Here's how the part is built. I have some questions about the finished solid (model axes, mm). A direction names the side the tool comes from. Coordinates: 2 decimals unless noted, no trailing zeros. Order: outer loops, then holes, each group sorted by start corner. A loop starts at its lowest first (then second) coordinate and runs counter-clockwise, first axis right, second up. Notation, with made-up numbers: (-13, 63) - (-1, 63) arc R23 ccw to (-1, 82) - close; hole circle Ø2 at (-33, 86). An arc over 180 degrees is marked (long way). Answer in a Markdown table with one row per item. Add a question column.
Item 1: Thinking about a two-plate mould opening in X: for faces 3 (the flat face through (-13, -2, 0)), 4 (the cylindrical face through (-46.344, -13.041, 49.042)), 5 (the cylindrical face through (-12.55, 7.497, 36.005)), which applies, +X half, -X half, draft (parallel to the pull), parting line (faces both ways), or undercut?
Item 2: On a 3-axis mill with a long thin cutter (end or side, diameter ignored), from which of +Z, -Z, +X, -X, +Y, -Y can I reach the whole of each face in a straight line? I mean faces 1 (the flat face through (-47.77, 5, 26)), 2 (the flat face through (-13, -5, 6)). Say none if no direction works.
Item 3: I want a section at C-C (x = -3.5). Please give me the cut outline in (y, z).
Item 4: I want a section at D-D (y = 3). Please give me the cut outline in (x, z).
Item 5: If I drill on line 1 along X through (y, z) = (-9.25, 49.5); line 2 along Z through (x, y) = (-22, -12.25); line 3 along Y through (x, z) = (-42.5, 47), over which ranges is the centre line in solid material (lowest first)? Write a range as from..to.
Item 6: I want a section at A-A (z = 11). Please give me the cut outline in (x, y), plus the area to 3 significant figures.
Item 7: Will these pins go through, and if not, where does the flat tip stop? pin 1 Ø1.5 at (y, z) = (3, 34) entering from -X; pin 2 Ø6 at (x, y) = (-42.77, -9.54) entering from -Z; pin 3 Ø10 at (x, z) = (4, 36) entering from -Y.
Item 8: I want a section at B-B (y = -10.5). Please give me the cut outline in (x, z).
```python
from build123d import *

# Parameters (mm, degrees)
SKETCH_1_W          = 70
SKETCH_1_H          = 25
SKETCH_1_R          = 2.5
EXTRUDE_1_DEPTH     = 52
FILLET_6_R          = 5
FILLET_7_R          = 5
SKETCH_2_W          = 40
SKETCH_2_H          = 19
CUT_EXTRUDE_2_DEPTH = 89.405565637
SKETCH_3_R          = 5
CUT_EXTRUDE_3_DEPTH = 75.906573986


with BuildPart() as part:
    # 草图1 → 凸台-拉伸1 (new body)
    with BuildSketch(Plane.XY):
        with Locations((-12.770229498, -2.044553468)):
            Rectangle(SKETCH_1_W, SKETCH_1_H)
        with Locations(Location((-42.770229498, -9.544553468, 0), (0, 0, 180))):
            Circle(SKETCH_1_R, mode=Mode.SUBTRACT)
        with Locations(Location((17.229770502, -9.544553468, 0), (0, 0, 180))):
            Circle(SKETCH_1_R, mode=Mode.SUBTRACT)
    extrude(amount=EXTRUDE_1_DEPTH)

    # 圆角6
    fillet_6_edges = [part.edges().sort_by_distance(p)[0] for p in [
        (-47.770229498, -14.544553468, 26),
    ]]
    fillet(fillet_6_edges, radius=FILLET_6_R)

    # 圆角7
    fillet_7_edges = [part.edges().sort_by_distance(p)[0] for p in [
        (22.229770502, -14.544553468, 26),
    ]]
    fillet(fillet_7_edges, radius=FILLET_7_R)

    # 草图2 → 切除-拉伸2 (cut, through all)
    with BuildSketch(Plane.ZY.offset(47.770229498)):
        with Locations((26, -5.044553468)):
            Rectangle(SKETCH_2_W, SKETCH_2_H)
    extrude(amount=-CUT_EXTRUDE_2_DEPTH, mode=Mode.SUBTRACT)

    # 草图3 → 切除-拉伸3 (cut, through all)
    with BuildSketch(Plane(origin=(0, 10.455446532, 0), x_dir=(1, 0, 0), z_dir=(0, 1, 0))):
        with Locations(Location((-12.770229498, -11, 0), (0, 0, 180))):
            Circle(SKETCH_3_R)
        with Locations(Location((-12.770229498, -41, 0), (0, 0, 270))):
            Circle(SKETCH_3_R)
    extrude(amount=-CUT_EXTRUDE_3_DEPTH, mode=Mode.SUBTRACT)


solid = part.part
```
Values follow:
| question | item | result |
|---|---|---|
| 1 | face 3 | draft |
| 1 | face 4 | -X half |
| 1 | face 5 | undercut |
| 2 | face 1 | +Z, -Z, -X, +Y, -Y |
| 2 | face 2 | +X, -X, -Y |
| 3 | outline | (-14.54, 0) - (10.46, 0) - (10.46, 52) - (-14.54, 52) - (-14.54, 46) - (4.46, 46) - (4.46, 6) - (-14.54, 6) - close |
| 4 | outline | (-47.77, 0) - (22.23, 0) - (22.23, 6) - (-47.77, 6) - close; (-47.77, 46) - (22.23, 46) - (22.23, 52) - (-47.77, 52) - close |
| 5 | line 1 | x = -47.77..-45.25, -40.29..14.75, 19.71..22.23 |
| 5 | line 2 | z = 0..6, 46..52 |
| 5 | line 3 | y = -14.54..-12.03, -7.06..10.46 |
| 6 | outline | (-47.77, 4.46) - (-17.77, 4.46) - (-17.77, 10.46) - (-47.77, 10.46) - close; (-7.77, 4.46) - (22.23, 4.46) - (22.23, 10.46) - (-7.77, 10.46) - close |
| 6 | area | 360 mm^2 |
| 7 | pin 1 | passes through |
| 7 | pin 2 | stops at z = 0 |
| 7 | pin 3 | stops at y = 4.46 |
| 8 | outline | (-47.68, 0) - (-45.08, 0) - (-45.08, 6) - (-47.68, 6) - close; (-47.68, 46) - (-45.08, 46) - (-45.08, 52) - (-47.68, 52) - close; (-40.46, 0) - (14.92, 0) - (14.92, 6) - (-40.46, 6) - close; (-40.46, 46) - (14.92, 46) - (14.92, 52) - (-40.46, 52) - close; (19.54, 0) - (22.14, 0) - (22.14, 6) - (19.54, 6) - close; (19.54, 46) - (22.14, 46) - (22.14, 52) - (19.54, 52) - close |
